from build123d import *

# Parameters (mm, degrees)
SKETCH2_R               = 26.5
BOSS_EXTRUDE1_DEPTH     = 1.6
CUT_EXTRUDE2_DEPTH      = 38.510798445
CUT_EXTRUDE2_DEPTH_BACK = 38.510798445
SKETCH1_R               = 2.5
SKETCH3_R               = 7.5
BOSS_EXTRUDE2_DEPTH     = 6.5
F_5_0MM_DOWEL_HOLE2_D   = 5


with BuildPart() as part:
    # Sketch2 → Boss-Extrude1 (new, symmetric)
    with BuildSketch(Plane(origin=(0, 0, 0), x_dir=(1, 0, 0), z_dir=(0, 1, 0))):
        with Locations(Location((0, 0, 0), (0, 0, 90))):
            Circle(SKETCH2_R)
    extrude(amount=BOSS_EXTRUDE1_DEPTH, both=True)

    # Sketch1 → Cut-Extrude2 (cut, two sides: drawn at the far end of the back side and taken through both)
    with BuildSketch(Plane(origin=(0, 0, 0), x_dir=(1, 0, 0), z_dir=(0, 1, 0)).offset(-CUT_EXTRUDE2_DEPTH_BACK)):
        with Locations((0, 26.5)):
            Circle(SKETCH1_R)
        with Locations((6.341865104, 25.729958162)):
            Circle(SKETCH1_R)
        with Locations((12.315164059, 23.46458468)):
            Circle(SKETCH1_R)
        with Locations((17.572750443, 19.835534827)):
            Circle(SKETCH1_R)
        with Locations((21.809072446, 15.053715788)):
            Circle(SKETCH1_R)
        with Locations((24.777930431, 9.397029507)):
            Circle(SKETCH1_R)
        with Locations((26.306785164, 3.194222027)):
            Circle(SKETCH1_R)
        with Locations((26.306785164, -3.194222027)):
            Circle(SKETCH1_R)
        with Locations((24.777930431, -9.397029507)):
            Circle(SKETCH1_R)
        with Locations((21.809072446, -15.053715788)):
            Circle(SKETCH1_R)
        with Locations((17.572750443, -19.835534827)):
            Circle(SKETCH1_R)
        with Locations((12.315164059, -23.46458468)):
            Circle(SKETCH1_R)
        with Locations((6.341865104, -25.729958162)):
            Circle(SKETCH1_R)
        with Locations((0, -26.5)):
            Circle(SKETCH1_R)
        with Locations((-6.341865104, -25.729958162)):
            Circle(SKETCH1_R)
        with Locations((-12.315164059, -23.46458468)):
            Circle(SKETCH1_R)
        with Locations((-17.572750443, -19.835534827)):
            Circle(SKETCH1_R)
        with Locations((-21.809072446, -15.053715788)):
            Circle(SKETCH1_R)
        with Locations((-24.777930431, -9.397029507)):
            Circle(SKETCH1_R)
        with Locations((-26.306785164, -3.194222027)):
            Circle(SKETCH1_R)
        with Locations((-26.306785164, 3.194222027)):
            Circle(SKETCH1_R)
        with Locations((-24.777930431, 9.397029507)):
            Circle(SKETCH1_R)
        with Locations((-21.809072446, 15.053715788)):
            Circle(SKETCH1_R)
        with Locations((-17.572750443, 19.835534827)):
            Circle(SKETCH1_R)
        with Locations((-12.315164059, 23.46458468)):
            Circle(SKETCH1_R)
        with Locations((-6.341865104, 25.729958162)):
            Circle(SKETCH1_R)
    extrude(amount=CUT_EXTRUDE2_DEPTH + CUT_EXTRUDE2_DEPTH_BACK, mode=Mode.SUBTRACT)

    # Sketch3 → Boss-Extrude2 (add, symmetric)
    with BuildSketch(Plane(origin=(0, 0, 0), x_dir=(1, 0, 0), z_dir=(0, 1, 0))):
        with Locations(Location((0, 0, 0), (0, 0, 90))):
            Circle(SKETCH3_R)
    extrude(amount=BOSS_EXTRUDE2_DEPTH, both=True)

    # Ø5.0mm Dowel Hole2 (through all)
    with Locations(Plane(origin=(0, 6.5, 0), x_dir=(1, 0, 0), z_dir=(0, 1, 0))):
        with Locations((0, 0)):
            Hole(F_5_0MM_DOWEL_HOLE2_D / 2)


solid = part.part
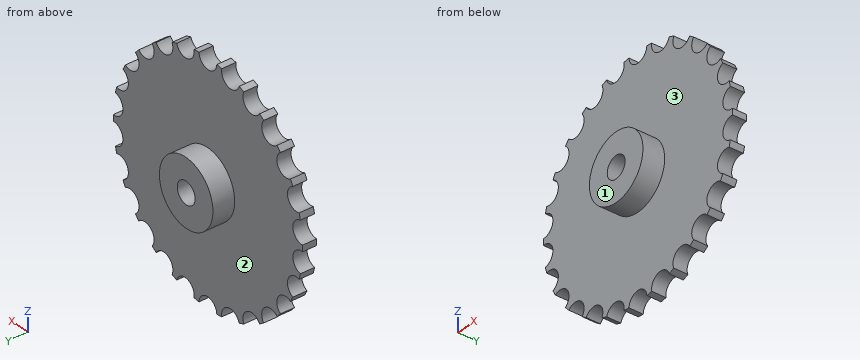
The listing builds one solid part. Answer for the finished solid, in the listing's coordinates (mm). Face numbers are marked on the shaded views. A direction names the side the tool comes from. Round coordinates to 2 decimals unless told otherwise and drop trailing zeros. Write each loop counter-clockwise with the first axis right and the second up, starting at its lowest first coordinate (ties: lowest second). Pieces come first, ordered by that corner, then holes. Notation, with made-up numbers: M -39.5,36.5 L 9.5,36.5 A21 ccw 9.5,62.5 Z; hole C -4,35.5 d8. An arc over 180 degrees is marked long. Write each question's results on one line, items separated by ' | '. Start each with the question number.
Item 1: Find section D-D on x = -12. Write down the section's boundary in (y, z), and give its area (3 significant figures).
Item 2: Which of the six approach directions +Z, -Z, +X, -X, +Y, -Y give full straight-line access (tool end or side, diameter ignored) to the marked faces 1, 2 and 3?
Item 3: Straight lines are drawn through the part: probe 1 along Z at (x, y) = (-23.5, 0.25); probe 2 along Y at (x, z) = (13.5, -2.5); probe 3 along X at (y, z) = (-0.25, -14.5). For each, find the intervals that lie inside material, in ascending order.
Item 4: Find section C-C on y = 3.5. Write down the section's boundary in (x, z).
Item 5: Given pin 1 Ø5 at (y, z) = (1.5, 7) entering from +X; pin 2 Ø6.5 at (x, z) = (0, 0) entering from +Y; pin 3 Ø1.5 at (x, y) = (-12, 4) entering from +Z; pin 4 Ø2 at (x, y) = (-16.5, -2) entering from -Z, each flat-ended and moving along its own axis, determine where each tip first touches the part or whether it passes through.
Item 6: Find section B-B on z = 0. Write down the section's boundary in (x, y).
Item 7: Find section A-A on x = 0. Write down the section's boundary in (y, z).
Answer block:
1) outline: M -1.6,-20.98 L 1.6,-20.98 L 1.6,20.98 L -1.6,20.98 Z | area: 134 mm²
2) face 1: +Z, -Z, +X, -X, -Y | face 2: +Y | face 3: -Y
3) probe 1: z = -12.25 to -11.55, -7.25 to 7.25, 11.55 to 12.25 | probe 2: y = -1.6 to 1.6 | probe 3: x = -19.37 to 19.37
4) outline: C 0,0 d15; hole C 0,0 d5
5) pin 1: stops at x = 25.89 | pin 2: stops at y = 6.5 | pin 3: passes through | pin 4: stops at z = -21.43
6) outline: M -26.5,-1.6 L -7.5,-1.6 L -7.5,-6.5 L -2.5,-6.5 L -2.5,6.5 L -7.5,6.5 L -7.5,1.6 L -26.5,1.6 Z; M 2.5,-6.5 L 7.5,-6.5 L 7.5,-1.6 L 26.5,-1.6 L 26.5,1.6 L 7.5,1.6 L 7.5,6.5 L 2.5,6.5 Z
7) outline: M -6.5,-7.5 L -1.6,-7.5 L -1.6,-24 L 1.6,-24 L 1.6,-7.5 L 6.5,-7.5 L 6.5,-2.5 L -6.5,-2.5 Z; M -6.5,2.5 L 6.5,2.5 L 6.5,7.5 L 1.6,7.5 L 1.6,24 L -1.6,24 L -1.6,7.5 L -6.5,7.5 Z
